Part model, mm, in its own coordinate system. Round coordinates to 2 decimals unless told otherwise and drop trailing zeros. Write each loop counter-clockwise with the first axis right and the second up, starting at its lowest first coordinate (ties: lowest second). Pieces come first, ordered by that corner, then holes. Notation, with made-up numbers: M 40,27.5 L 78,27.5 A29 ccw 78,52.5 Z; hole C 34,-25 d11. An arc over 180 degrees is marked long. Use a Markdown table: item, result. Add a question column.
1) Drop flat-ended pins along their axis: P1, Ø3, axis at x = -4.76, y = 12.7, coming from the +Z side (3 decimals); P2, Ø8, axis at x = 8.5, z = -1, coming from the -Y side; P3, Ø1.6, axis at x = 11.5, z = 3.5, coming from the +Y side. Give the stop position or say it passes through.
2) Slice it at B-B on y = 513.5. Write the cut outline in (x, z) (3 decimals).
3) Wall check: probe 1 along Y at (x, z) = (0, 10.5); probe 2 along Z at (x, y) = (3, 69) (3 decimals). Give the ranges that are in metal, low to high.
4) Slice it at A-A on z = -1.5. Write the cut outline in (x, y) (3 decimals).
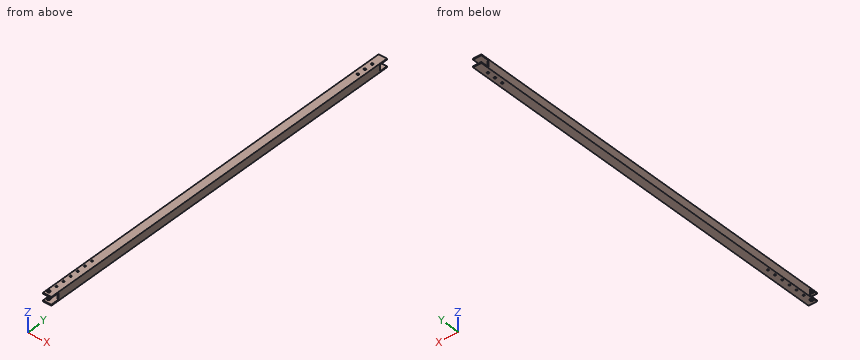
```python
from build123d import *

# Parameters (mm, degrees)
SKETCH1_W                       = 25.4
SKETCH1_H                       = 25.4
SKETCH1_W_2                     = 19.05
SKETCH1_H_2                     = 19.05
BOSS_EXTRUDE1_DEPTH             = 1143
F_10_CLEARANCE_HOLE1_D          = 5.1054
F_10_CLEARANCE_HOLE2_AT_2_COUNT = 2
F_10_CLEARANCE_HOLE2_AT_2_PITCH = 50.8
F_10_CLEARANCE_HOLE2_AT_3_COUNT = 2
F_10_CLEARANCE_HOLE2_AT_3_PITCH = 25.4
SKETCH6_W                       = 25.4
SKETCH6_H                       = 3.175
BOSS_EXTRUDE2_DEPTH             = 25.4
SKETCH7_W                       = 25.4
SKETCH7_H                       = 3.175
BOSS_EXTRUDE3_DEPTH             = 25.4
F_3_8_0_375_DIAMETER_HOLE2_D    = 9.525


with BuildPart() as part:
    # Sketch1 → Boss-Extrude1 (new body)
    with BuildSketch(Plane(origin=(0, 0, 0), x_dir=(1, 0, 0), z_dir=(0, 1, 0))):
        Rectangle(SKETCH1_W, SKETCH1_H)
        Rectangle(SKETCH1_W_2, SKETCH1_H_2, mode=Mode.SUBTRACT)
    extrude(amount=BOSS_EXTRUDE1_DEPTH)

    # #10 Clearance Hole1 (through all)
    with Locations(Plane.XY.offset(12.7)):
        with Locations((-4.7625, 114.3), (-4.7625, 63.5), (-4.7625, 38.1), (-4.7625, 12.7), (-4.7625, 139.7), (-4.7625, 88.9)):
            Hole(F_10_CLEARANCE_HOLE1_D / 2)

    # Sketch5 → #10 Clearance Hole2 (revolve, cut)
    with BuildSketch(Plane(origin=(0, 1130.3, 12.7), x_dir=(0, -1, 0), z_dir=(1, 0, 0))):
        Polygon((0, 0), (0, 25.4), (3.1877, 25.4), (2.5527, 24.765), (2.5527, 0.635), (3.1877, 0), align=None)
    f_10_clearance_hole2 = revolve(axis=Axis((0, 1130.3, 19.05), (0, 0, -1)), mode=Mode.SUBTRACT)

    # #10 Clearance Hole2 at 2: #10 Clearance Hole2 ×2
    with Locations(*[(0, -i * F_10_CLEARANCE_HOLE2_AT_2_PITCH, 0) for i in range(1, F_10_CLEARANCE_HOLE2_AT_2_COUNT)]):
        add(f_10_clearance_hole2, mode=Mode.SUBTRACT)

    # #10 Clearance Hole2 at 3: #10 Clearance Hole2 ×2
    with Locations(*[(0, -i * F_10_CLEARANCE_HOLE2_AT_3_PITCH, 0) for i in range(1, F_10_CLEARANCE_HOLE2_AT_3_COUNT)]):
        add(f_10_clearance_hole2, mode=Mode.SUBTRACT)

    # Sketch6 → Boss-Extrude2 (add)
    with BuildSketch(Plane(origin=(0, 1143, 0), x_dir=(1, 0, 0), z_dir=(0, 1, 0))):
        with Locations((0, 11.1125)):
            Rectangle(SKETCH6_W, SKETCH6_H)
        with Locations((0, -11.1125)):
            Rectangle(SKETCH6_W, SKETCH6_H)
    extrude(amount=BOSS_EXTRUDE2_DEPTH)

    # Sketch7 → Boss-Extrude3 (add)
    with BuildSketch(Plane.XZ):
        with Locations((0, -11.1125)):
            Rectangle(SKETCH7_W, SKETCH7_H)
        with Locations((0, 11.1125)):
            Rectangle(SKETCH7_W, SKETCH7_H)
    extrude(amount=BOSS_EXTRUDE3_DEPTH)

    # 3/8 (0.375) Diameter Hole2 (through all)
    with Locations(Plane.XY.offset(12.7)):
        with Locations((-6.35, -12.7)):
            Hole(F_3_8_0_375_DIAMETER_HOLE2_D / 2)


solid = part.part
```
Entries:
| question | item | result |
|---|---|---|
| 1 | P1 | passes through |
| 1 | P2 | stops at y = 0 |
| 1 | P3 | stops at y = 1143 |
| 2 | outline | M -12.7,-12.7 L 12.7,-12.7 L 12.7,12.7 L -12.7,12.7 Z; hole M -9.525,-9.525 L 9.525,-9.525 L 9.525,9.525 L -9.525,9.525 Z |
| 3 | probe 1 | y = -25.4 to 1076.95, 1082.05 to 1102.35, 1107.45 to 1127.75, 1132.85 to 1168.4 |
| 3 | probe 2 | z = -12.7 to -9.525, 9.525 to 12.7 |
| 4 | outline | M -12.7,0 L -9.525,0 L -9.525,1143 L -12.7,1143 Z; M 9.525,0 L 12.7,0 L 12.7,1143 L 9.525,1143 Z |
